Design review of the part built by this model. Coordinates are the model's own, in mm. Round coordinates to 2 decimals unless told otherwise and drop trailing zeros. Loops run counter-clockwise (first coordinate to the right, second up) from the corner with the lowest first, then second, coordinate; pieces in that order, holes last. Notation, with made-up numbers: (79.25, 84) - (85.25, 84) arc R17 ccw to (85.25, 113) - close; hole circle Ø4 at (15.25, 13). An arc over 180 degrees is marked (long way). Answer as CSV lines item,"result". Start each with the question number.
(1) For P1, Ø12, axis at y = -287, z = -134, coming from the +X side; P2, Ø5, axis at x = 206, z = -132, coming from the +Y side; P3, Ø10, axis at x = 30.5, z = -150, coming from the +Y side, all flat-tipped, find the tip position at first contact; note any pin that passes through.
(2) Consider section B-B (x = 28.5). Give the boundary of the cut face in (y, z).
(3) Wall thickness on L1, parallel to X at y = -285, z = -143; L2, parallel to Y at x = -65.5, z = -161.5; L3, parallel to Y at x = 210.5, z = -106.5: over which ranges is each line inside the solid? List them lowest first.
(4) Consider section A-A (x = -207). Give the boundary of the cut face in (y, z).
from build123d import *

# Parameters (mm, degrees)
F1_DEPTH = 25.4
F3_DEPTH = 31.75
F5_DEPTH = 25.4
F6_W     = 25.4
F6_H     = 270.2104524793
F7_DEPTH = 508


with BuildPart() as f1:
    # F0 (on Right) → F1 (new body)
    with BuildSketch(Plane.YZ):
        Polygon((27.3959822953, -102.7910036798), (27.3959822953, 85.8886760547), (-43.5209119504, 143.3160446986), (-242.814470184, -102.7910036798), align=None)
    extrude(amount=F1_DEPTH)

    # F6 (on face) → F7 (cut)
    with BuildSketch(Plane(origin=(0, 0, -102.7910036798), x_dir=(1, 0, 0), z_dir=(0, 0, -1))):
        with Locations((12.7, 107.7092439444)):
            Rectangle(F6_W, F6_H)
    extrude(amount=-F7_DEPTH, mode=Mode.SUBTRACT)


with BuildPart() as f3:
    # F2 (on face) → F3 (new body)
    with BuildSketch(Plane(origin=(0, -96.3768318043, 78.044419565), x_dir=(1, 0, 0), z_dir=(0, -0.7771459615, 0.629320391))):
        with BuildLine():
            Line((0, -232.6917107126), (-255.0972491243, -232.6917107126))
            ThreePointArc((-255.0972491243, -232.6917107126), (12.7, -330.742311978), (280.4972491243, -232.6917107126))
            Line((280.4972491243, -232.6917107126), (25.4, -232.6917107126))
            Line((25.4, -232.6917107126), (12.7, -232.6917107126))
            Line((12.7, -232.6917107126), (0, -232.6917107126))
        make_face()
    extrude(amount=F3_DEPTH)

    # F4 (on face) → F5 (cut)
    with BuildSketch(Plane(origin=(0, 0, -102.7910036798), x_dir=(1, 0, 0), z_dir=(0, 0, -1))):
        Polygon((0, 242.814470184), (12.7, 242.814470184), (25.4, 242.814470184), (293.8941717148, 242.814470184), (293.8941717148, 285.4833602905), (-263.440400362, 285.4833602905), (-263.440400362, 242.814470184), align=None)
    extrude(amount=-F5_DEPTH, mode=Mode.SUBTRACT)


solid = f3.part
Determined:
1,P1,"stops at x = 213.75"
1,P2,"stops at y = -264.44"
1,P3,"stops at y = -276.99"
2,outline,"(-329, -158.78) - (-304.33, -178.76) - (-242.81, -102.79) - (-283.67, -102.79) - close"
3,L1,"x = -165.54 to 190.94"
3,L2,"y = -314.3 to -290.36"
3,L3,"y = -286.67 to -245.82"
4,outline,"(-289.56, -110.07) - (-264.89, -130.05) - (-242.81, -102.79) - (-283.67, -102.79) - close"
